Build history of the part. All positions in model axes, mm. A direction names the side the tool comes from. Coordinates: 2 decimals unless noted, no trailing zeros. Write each loop counter-clockwise with the first axis right and the second up, starting at its lowest first coordinate (ties: lowest second). Pieces come first, ordered by that corner, then holes.
Autodesk Inventor part; units mm, degrees
ref_plane "YZ Plane" through (0, 0, 0) normal (1, 0, 0) x (0, 1, 0)
ref_plane "XZ Plane" through (0, 0, 0) normal (0, 1, 0) x (-1, 0, 0)
ref_plane "XY Plane" through (0, 0, 0) normal (0, 0, 1) x (1, 0, 0)
sketch "Szkic1" plane through (0, 0, 0) normal (0, 1, 0) x (-1, 0, 0)
  line L0 (-3.4059, 22.6049) -> (16.5941, 22.6049)
  line L1 (16.5941, 22.6049) -> (16.5941, -8.3951)
  line L2 (16.5941, -8.3951) -> (-3.4059, -8.3951)
  line L3 (-3.4059, -8.3951) -> (-3.4059, 22.6049)
  point P0 (0, 0)
  dimension "d0" = 20
  dimension "d1" = 31
extrude "Wyciągnięcie proste1" add sketch "Szkic1" along normal blind 4
sketch "Szkic2" plane through (0, 4, 0) normal (0, 1, 0) x (1, 0, 0)
  line L0 (-16.5941, 8.3951) -> (-16.5941, -22.6049)
  line L1 (-16.5941, -22.6049) -> (3.4059, -22.6049)
  line L2 (-16.5941, -22.6049) -> (3.4059, -22.6049)
  line L3 (3.4059, -22.6049) -> (3.4059, 8.3951)
  line L4 (3.4059, -22.6049) -> (3.4059, 8.3951)
  line L5 (3.4059, 8.3951) -> (-16.5941, 8.3951)
  line L6 (3.4059, 8.3951) -> (-16.5941, 8.3951)
  line L7 (-16.5941, 8.3951) -> (-16.5941, -22.6049)
  line L8 (-16.5941, -12.6049) -> (3.4059, -12.6049)
  line L9 (-16.5941, -1.6049) -> (3.4059, -1.6049)
  point P0 (0, 0)
  point P1 (-6.5941, -18.6049)
  point P2 (-6.5941, 4.3951)
  dimension "d4" = 10
  dimension "d5" = 10
  dimension "d6" = 10
  dimension "d7" = 10
  dimension "d8" = 4
  dimension "d9" = 4
extrude "Wyciągnięcie proste2" add sketch "Szkic2" along normal blind 4 contours L9 L3 L8 L0
fillet "Zaokrąglenie1" radius 4 4 edges at (3.4059, 2, -8.3951) (-16.5941, 2, -8.3951) (3.4059, 2, 22.6049) (-16.5941, 2, 22.6049)
hole "Otwór1" at (-6.5941, 4, 18.6049) at (-6.5941, 4, -4.3951) direction (0, -1, 0) diameter 4.15 end through all
fillet "Zaokrąglenie2" radius 1 4 edges at (3.4059, 6, 1.6049) (3.4059, 6, 12.6049) (-16.5941, 6, 1.6049) (-16.5941, 6, 12.6049)
chamfer "Faza1" distance 1 angle 45 2 edges at (-6.5941, 4, 16.5299) (-6.5941, 4, -6.4701)
properties part number "3DP_ABS_Z_Axis_Endstop_Mount"
1. Flat gauge pins, fed straight in: pin 1 (5.5 mm diameter, centred on x = -10.5, z = -4.5, fed in from +Y); pin 2 (2 mm diameter, centred on x = -2.5, y = 6, fed in from +Z); pin 3 (3.5 mm diameter, centred on x = -6.59, z = 18.6, fed in from +Y); pin 4 (2 mm diameter, centred on x = -3, y = 6, fed in from -Z). Where does each tip first touch, or does it go through?
Computed values:
pin 1: stops at y = 4
pin 2: stops at z = 12.6
pin 3: passes through
pin 4: stops at z = 1.6
2. Saw through at A-A on y = 6.75. List the corners of the cut face in (x, z), plus the area to 3 significant figures.
Computed values:
outline: (-16.59, 2.6) arc R1 ccw to (-15.59, 1.6) - (2.41, 1.6) arc R1 ccw to (3.41, 2.6) - (3.41, 11.6) arc R1 ccw to (2.41, 12.6) - (-15.59, 12.6) arc R1 ccw to (-16.59, 11.6) - close
area: 219 mm2
3. Mould opens along X. For faces 4 (the face through (2.27, 2.03, -7.19)), 5 (the face through (-4, 4, 16)), 6 (the face through (-8.344, 1.479, 19.72)) say: +X half, -X half, draft (parallel to the pull), parting line (faces both ways), or undercut.
Computed values:
face 4: +X half
face 5: draft
face 6: undercut
4. Saw through at D-D on z = 13. List the corners of the cut face in (x, y), plus the area to 3 significant figures.
Computed values:
outline: (-16.59, 0) - (3.41, 0) - (3.41, 4) - (-16.59, 4) - close
area: 80.0 mm2
5. Saw through at B-B on x = -10. List the corners of the cut face in (y, z), plus the area to 3 significant figures.
Computed values:
outline: (0, -8.4) - (4, -8.4) - (4, 1.6) - (8, 1.6) - (8, 12.6) - (4, 12.6) - (4, 22.6) - (0, 22.6) - close
area: 168 mm2
6. Probe line 1 along Z through (x, y) = (-7.5, 3.25); line 2 along Z through (x, y) = (-5.25, 7.5); line 3 along X through (y, z) = (2, -4.5). List the from-to ranges inside material, lowest first.
Computed values:
line 1: z = -8.4 to -6.54, -2.25 to 16.46, 20.75 to 22.6
line 2: z = 1.6 to 12.6
line 3: x = -16.59 to -8.67, -4.52 to 3.4
7. 3-axis set-ups, long thin cutter, end or side, ignore diameter. For faces 1 (the face through (-16.309, 6.028, 12.304)), 2 (the face through (3.121, 6.028, 1.906)), 3 (the face through (-16.293, 6.028, 1.89)): which of +Z, -Z, +X, -X, +Y, -Y reach the whole face in a straight line?
Computed values:
face 1: +Z, -X, +Y
face 2: -Z, +X, +Y
face 3: -Z, -X, +Y
8. Saw through at C-C on y = 2. List the corners of the cut face in (x, z) (3 decimals), plus the area to 3 significant figures.
Computed values:
outline: (-16.594, -4.395) arc R4 ccw to (-12.594, -8.395) - (-0.594, -8.395) arc R4 ccw to (3.406, -4.395) - (3.406, 18.605) arc R4 ccw to (-0.594, 22.605) - (-12.594, 22.605) arc R4 ccw to (-16.594, 18.605) - close; hole circle Ø4.15 at (-6.594, -4.395); hole circle Ø4.15 at (-6.594, 18.605)
area: 579 mm2
